Check sheet for the modelled part. Datum: model origin and axes. Units: mm. Face numbers are marked on the shaded views. A direction names the side the tool comes from. Give positions to 0.01 mm unless a question says otherwise; leave off trailing zeros. Write each loop counter-clockwise with the first axis right and the second up, starting at its lowest first coordinate (ties: lowest second). Pieces come first, ordered by that corner, then holes. Notation, with made-up numbers: (-33.5, 82) -> (-22.5, 82) arc R30 cw to (-22.5, 116) -> close; hole circle Ø4 at (-31, 81.5). An arc over 180 degrees is marked (long way). Write each question's results on one line, items separated by ' | '. Start each with the question number.
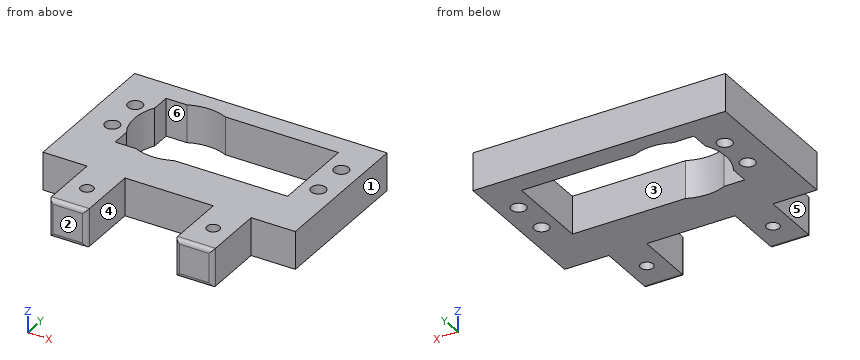
```python
from build123d import *

# Parameters (mm, degrees)
CROQUIS1_R              = 1.75
CROQUIS1_R_2            = 1.5
SALIENTE_EXTRUIR1_DEPTH = 9
REDONDEO1_R             = 1


with BuildPart() as part:
    # Croquis1 → Saliente-Extruir1 (new body)
    with BuildSketch(Plane.XY):
        Polygon((0, 36), (0, 0), (10.5, 0), (10.5, -15), (19.5, -15), (19.5, 0), (40.5, 0), (40.5, -15), (49.5, -15), (49.5, 0), (60, 0), (60, 36), align=None)
        with Locations((6.5, 16.5)):
            Circle(CROQUIS1_R, mode=Mode.SUBTRACT)
        with Locations((6.5, 25.5)):
            Circle(CROQUIS1_R, mode=Mode.SUBTRACT)
        with BuildLine():
            Line((10.5, 26.545268253), (10.5, 31))
            Line((10.5, 31), (15.417424305, 31))
            ThreePointArc((15.417424305, 31), (20, 32), (24.582575695, 31))
            Line((24.582575695, 31), (51.5, 31))
            Line((51.5, 31), (51.5, 11))
            Line((51.5, 11), (24.582575695, 11))
            ThreePointArc((24.582575695, 11), (20, 10), (15.417424305, 11))
            Line((15.417424305, 11), (10.5, 11))
            Line((10.5, 11), (10.5, 15.454731747))
            ThreePointArc((10.5, 15.454731747), (9, 21), (10.5, 26.545268253))
        make_face(mode=Mode.SUBTRACT)
        with Locations((55.5, 16.5)):
            Circle(CROQUIS1_R, mode=Mode.SUBTRACT)
        with Locations((55.5, 25.5)):
            Circle(CROQUIS1_R, mode=Mode.SUBTRACT)
        with Locations((15, -7.5)):
            Circle(CROQUIS1_R_2, mode=Mode.SUBTRACT)
        with Locations((45, -7.5)):
            Circle(CROQUIS1_R_2, mode=Mode.SUBTRACT)
    extrude(amount=SALIENTE_EXTRUIR1_DEPTH)

    # Redondeo1
    redondeo1_edges = [part.edges().sort_by_distance(p)[0] for p in [
        (45, -15, 0),
        (15, -15, 0),
        (49.5, -15, 4.5),
        (40.5, -15, 4.5),
        (19.5, -15, 4.5),
        (10.5, -15, 4.5),
        (15, -15, 9),
        (45, -15, 9),
    ]]
    fillet(redondeo1_edges, radius=REDONDEO1_R)


solid = part.part
```
Item 1: Section check C-C on z = 6.25. Count the separate pieces of the cut face and the enclosed holes in it, then the cut area to 3 significant figures.
Item 2: Section check B-B on x = 6.5. Record the boundary of the cut face in (y, z).
Item 3: Mould release check, pull along Y, two halves, no side actions. Record for the marked faces 1, 2 and 3: pulls with the +Y half, pulls with the -Y half, needs draft (parallel to the pull), parting line crosses it, or undercut.
Item 4: Depth check by flat-ended pin: pin 1 Ø4 at (y, z) = (-2.5, 5.5) entering from -X; pin 2 Ø4.5 at (x, z) = (55.5, 4.5) entering from -Y; pin 3 Ø2.5 at (y, z) = (-3.5, 3.5) entering from +X; pin 4 Ø2 at (x, y) = (55.5, 16.5) entering from -Z. Enter the tip coordinate at first touch or a pass-through.
Item 5: Section check A-A on y = -7.5. Record the boundary of the cut face in (x, z).
Item 6: Set-up check for the marked faces 4, 5 and 6: record each of +Z, -Z, +X, -X, +Y, -Y from which the full face is reachable in a straight line by a thin tool's end or side.
Item 7: Section check D-D on x = 27. Record the boundary of the cut face in (y, z), then the cut area to 3 significant figures.
Item 8: Thickness scan on probe 1 along Y at (x, z) = (45, 5); probe 2 along Y at (x, z) = (6.5, 5.75); probe 3 along Y at (x, z) = (12, 4). Record the ranges inside material, lowest first. Write a range as from..to.
Check sheet entries:
1) separate pieces: 1 | enclosed holes: 7 | area: 1,530 mm^2
2) outline: (0, 0) -> (14.75, 0) -> (14.75, 9) -> (0, 9) -> close; (18.25, 0) -> (23.75, 0) -> (23.75, 9) -> (18.25, 9) -> close; (27.25, 0) -> (36, 0) -> (36, 9) -> (27.25, 9) -> close
3) face 1: needs draft | face 2: pulls with the -Y half | face 3: undercut
4) pin 1: stops at x = 10.5 | pin 2: stops at y = 0 | pin 3: stops at x = 49.5 | pin 4: passes through
5) outline: (10.5, 0) -> (13.5, 0) -> (13.5, 9) -> (10.5, 9) -> close; (16.5, 0) -> (19.5, 0) -> (19.5, 9) -> (16.5, 9) -> close; (40.5, 0) -> (43.5, 0) -> (43.5, 9) -> (40.5, 9) -> close; (46.5, 0) -> (49.5, 0) -> (49.5, 9) -> (46.5, 9) -> close
6) face 4: +Z, -Z, -Y | face 5: +Z, -Z, -X, -Y | face 6: +Z, -Z
7) outline: (0, 0) -> (11, 0) -> (11, 9) -> (0, 9) -> close; (31, 0) -> (36, 0) -> (36, 9) -> (31, 9) -> close | area: 144 mm^2
8) probe 1: y = -15..-9, -6..11, 31..36 | probe 2: y = 0..14.75, 18.25..23.75, 27.25..36 | probe 3: y = -15..11, 31..36
